```python
from build123d import *

# Parameters (mm, degrees)
F1_DEPTH = 9
F3_DEPTH = 21


with BuildPart() as f1:
    # F0 (on Top) → F1 (new body)
    with BuildSketch(Plane.XY):
        with BuildLine():
            Line((5.692772, 19.450301), (-3.510716, 29.955687))
            Line((-3.510716, 29.955687), (-54.510716, 29.955687))
            ThreePointArc((-54.510716, 29.955687), (-69.499634, 15.532184), (-55.66286, 0))
            Line((-55.66286, 0), (-3.788572, 0))
            Line((-3.788572, 0), (5.692772, 9.250754))
            Line((5.692772, 9.250754), (5.692772, 19.450301))
        make_face()
    extrude(amount=F1_DEPTH)

    # F2 (on face) → F3 (join)
    with BuildSketch(Plane.XY.offset(9)):
        with BuildLine():
            Line((5.692772, 9.250754), (5.692772, 19.450301))
            Line((5.692772, 19.450301), (-36.291417, 19.450301))
            Line((-36.291417, 19.450301), (-36.291417, 29.955687))
            Line((-36.291417, 29.955687), (-54.510716, 29.955687))
            ThreePointArc((-54.510716, 29.955687), (-69.499634, 15.532184), (-55.66286, 0))
            Line((-55.66286, 0), (-36.291417, 0))
            Line((-36.291417, 0), (-36.291417, 9.250754))
            Line((-36.291417, 9.250754), (5.692772, 9.250754))
        make_face()
    extrude(amount=F3_DEPTH)


solid = f1.part
```
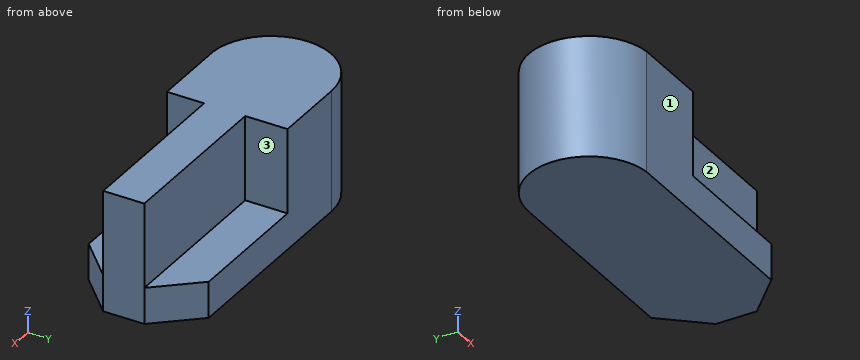
Work out the finished part from the listing and answer in its coordinate system (mm). Face numbers are marked on the shaded views. A direction names the side the tool comes from. Coordinates: 2 decimals unless noted, no trailing zeros. Write each loop counter-clockwise with the first axis right and the second up, starting at its lowest first coordinate (ties: lowest second). Pieces come first, ordered by that corner, then holes.
Q1. Find the intervals of material crossed by line 1 (Y direction, x = -11, z = 11.5); line 2 (Z direction, x = -3.5, y = 5.5); line 3 (X direction, y = 15.5, z = 7.25), in increasing order.
Q2. Each of these flat-tipped pins is pushed along its axis until it touches: pin 1 Ø10.5 at (x, z) = (-13, 20) entering from -Y; pin 2 Ø3 at (x, y) = (-19, 22.5) entering from +Z; pin 3 Ø10 at (y, z) = (23, 16.5) entering from -X. Where does it stop, or does it pass through?
Q3. A cutting plane is placed at B-B, the plane z = 18.75. Give the vertices of the cut face in (x, y).
Q4. A cutting plane is placed at D-D, the plane z = 4.75. Give the vertices of the cut face in (x, y), then the cut area to 3 significant figures.
Q5. Which of the six approach directions +Z, -Z, +X, -X, +Y, -Y give full straight-line access (tool end or side, diameter ignored) to the marked faces 1, 2 and 3?
Q6. A cutting plane is placed at A-A, the plane x = -31.5. Give the vertices of the cut face in (y, z), then the cut area to 3 significant figures.
Q7. A cutting plane is placed at C-C, the plane y = 22. Give the vertices of the cut face in (x, z), then the cut area to 3 significant figures.
Findings below:
1. line 1: y = 9.25 to 19.45
1. line 2: z = 0 to 9
1. line 3: x = -69.5 to 5.69
2. pin 1: stops at y = 9.25
2. pin 2: stops at z = 9
2. pin 3: stops at x = -69.2
3. outline: (-55.66, 0) - (-36.29, 0) - (-36.29, 9.25) - (5.69, 9.25) - (5.69, 19.45) - (-36.29, 19.45) - (-36.29, 29.96) - (-54.51, 29.96) arc R15 ccw to start
4. outline: (-55.66, 0) - (-3.79, 0) - (5.69, 9.25) - (5.69, 19.45) - (-3.51, 29.96) - (-54.51, 29.96) arc R15 ccw to start
4. area: 2,060 mm2
5. face 1: +Z, -Z, +X, -X, -Y
5. face 2: +Z, +X, -Y
5. face 3: +Z, +X, +Y
6. outline: (0, 0) - (29.96, 0) - (29.96, 9) - (19.45, 9) - (19.45, 30) - (9.25, 30) - (9.25, 9) - (0, 9) - close
6. area: 484 mm2
7. outline: (-67.75, 0) - (3.46, 0) - (3.46, 9) - (-36.29, 9) - (-36.29, 30) - (-67.75, 30) - close
7. area: 1,300 mm2
